Geometry: see drawing. Coordinates: mm, zero at the bounding-box minimum. A direction names the side the tool comes from. Coordinates: 2 decimals unless noted, no trailing zeros. Write each loop counter-clockwise with the first axis right and the second up, starting at its lowest first coordinate (ties: lowest second). Pieces come first, ordered by that corner, then holes.
1) Section query B-B (y = 28.75). Output: boundary loops of the cut face in (x, z).
2) Section query A-A (z = 79). Output: boundary loops of the cut face in (x, y), then the cut area to 3 significant figures.
3) Section query D-D (y = 15). Output: boundary loops of the cut face in (x, z).
4) Pin query (flat end, axial travel): pin 1 Ø11.5 at (x, z) = (27.5, 46) entering from +Y; pin 2 Ø10 at (x, y) = (30.5, 25.5) entering from +Z. Return the tip coordinate at first contact, or that it passes through.
5) Draft query along Z for the marked faces 3, 4 and 5. Return one class per face: pulls with the +Z half, pulls with the -Z half, needs draft (parallel to the pull), parting line crosses it, or undercut.
6) Section query C-C (x = 10). Output: boundary loops of the cut face in (y, z), then the cut area to 3 significant figures.
7) Set-up query: the marked faces 1 and 2. Return all of +Z, -Z, +X, -X, +Y, -Y with unobstructed straight access to the full face (end or side cutting, diameter ignored); none if empty.
8) Line query: L1, parallel to Z at x = 2.5, y = 41; L2, parallel to X at y = 48, z = 65; L3, parallel to Y at x = 22, z = 95.5. Output: solid intervals per line, ascending.
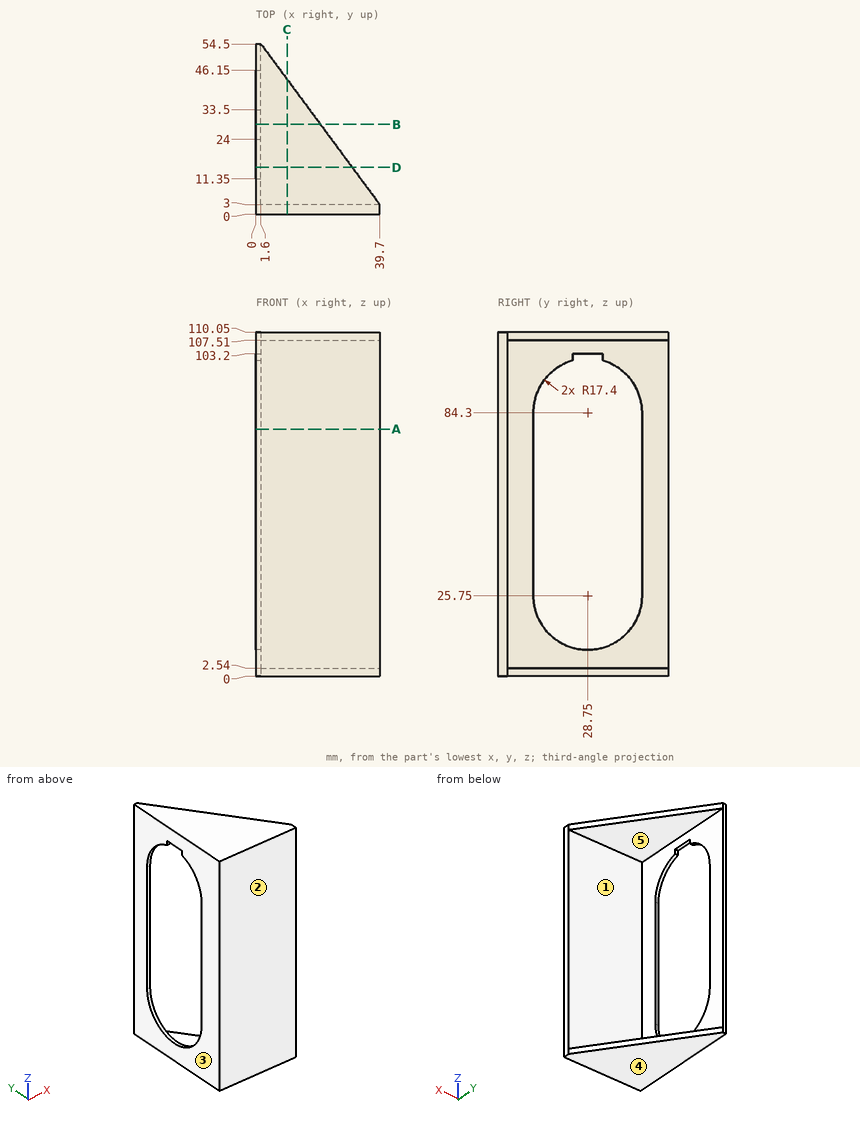
Answer:
1. outline: (0, 0) - (20.65, 0) - (20.65, 2.54) - (1.6, 2.54) - (1.6, 8.35) - (0, 8.35) - close; (0, 103.2) - (1.6, 103.2) - (1.6, 107.51) - (20.65, 107.51) - (20.65, 110.05) - (0, 110.05) - close
2. outline: (0, 0) - (39.7, 0) - (39.7, 3) - (1.6, 3) - (1.6, 11.35) - (0, 11.35) - close; (0, 46.15) - (1.6, 46.15) - (1.6, 54.5) - (0, 54.5) - close
2. area: 146 mm2
3. outline: (0, 0) - (30.82, 0) - (30.82, 2.54) - (1.6, 2.54) - (1.6, 15.09) - (0, 15.09) - close; (0, 94.96) - (1.6, 94.96) - (1.6, 107.51) - (30.82, 107.51) - (30.82, 110.05) - (0, 110.05) - close
4. pin 1: stops at y = 3
4. pin 2: passes through
5. face 3: needs draft
5. face 4: pulls with the -Z half
5. face 5: undercut
6. outline: (0, 0) - (43.15, 0) - (43.15, 2.54) - (3, 2.54) - (3, 107.51) - (43.15, 107.51) - (43.15, 110.05) - (0, 110.05) - close
6. area: 534 mm2
7. face 1: +X, +Y
7. face 2: +Z, -Z, +X, -X, -Y
8. L1: z = 0 to 2.54, 107.51 to 110.05
8. L2: x = 0 to 1.6
8. L3: y = 0 to 3
